Could you check a few things on this model? Use its own coordinates, in mm. Face numbers are marked on the shaded views. A direction names the side the tool comes from. Coordinates: 2 decimals unless noted, no trailing zeros. Loops run counter-clockwise (first coordinate to the right, second up) from the corner with the lowest first, then second, coordinate; pieces in that order, holes last. Notation, with made-up numbers: (55.25, 46) -> (96.25, 46) arc R35 ccw to (96.25, 85) -> close; hole circle Ø6 at (56.5, -32.5). An arc over 180 degrees is marked (long way). One line per question, with ' | ' between items.
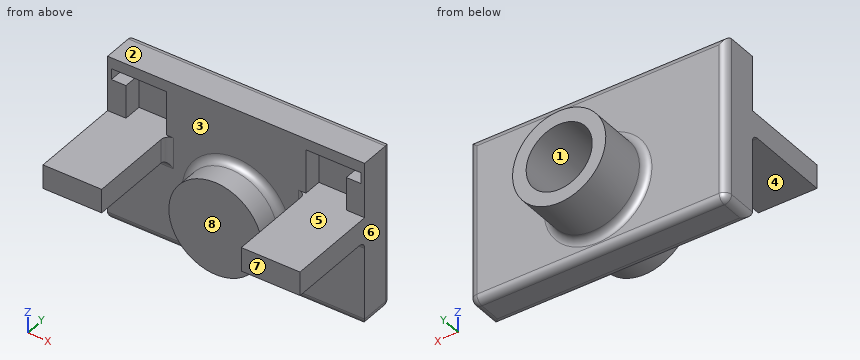
from build123d import *

# Parameters (mm, degrees)
SKETCH1_W           = 70
SKETCH1_H           = 45
BOSS_EXTRUDE1_DEPTH = 10
CUT_EXTRUDE1_DEPTH  = 5
FILLET1_R           = 2
SKETCH3_R           = 9
CUT_EXTRUDE3_DEPTH  = 25
BOSS_EXTRUDE2_START = 15
SKETCH5_R           = 12.7
SKETCH5_R_2         = 9
BOSS_EXTRUDE2_DEPTH = 15
FILLET2_R           = 2
SKETCH6_R           = 12.7
BOSS_EXTRUDE3_DEPTH = 8
FILLET3_R           = 2
SKETCH7_R           = 9
CUT_EXTRUDE4_DEPTH  = 5
SKETCH8_W           = 16
SKETCH8_H           = 6.5
BOSS_EXTRUDE4_DEPTH = 25
FILLET4_R           = 2


with BuildPart() as part:
    # Sketch1 → Boss-Extrude1 (new body)
    with BuildSketch(Plane(origin=(0, 0, 0), x_dir=(1, 0, 0), z_dir=(0, 1, 0))):
        with Locations((-1.479524439, -4.65323646)):
            Rectangle(SKETCH1_W, SKETCH1_H)
    extrude(amount=BOSS_EXTRUDE1_DEPTH)

    # Sketch2 → Cut-Extrude1 (cut)
    with BuildSketch(Plane.XZ):
        Polygon((28.520475561, 24.15323646), (17.520475561, 24.15323646), (17.520475561, 12.15323646), (28.520475561, 12.15323646), (28.520475561, 21.15323646), (32.520475561, 21.15323646), (32.520475561, 24.15323646), align=None)
        Polygon((-31.479524439, 21.15323646), (-35.479524439, 21.15323646), (-35.479524439, 24.15323646), (-31.479524439, 24.15323646), (-20.479524439, 24.15323646), (-20.479524439, 12.15323646), (-31.479524439, 12.15323646), align=None)
    extrude(amount=-CUT_EXTRUDE1_DEPTH, mode=Mode.SUBTRACT)

    # Fillet1
    fillet1_edges = [part.edges().sort_by_distance(p)[0] for p in [
        (33.520475561, 10, 4.65323646),
        (-1.479524439, 10, -17.84676354),
        (-36.479524439, 10, 4.65323646),
        (-1.479524439, 0, -17.84676354),
        (-36.479524439, 5, -17.84676354),
        (33.520475561, 5, -17.84676354),
        (-1.479524439, 10, 27.15323646),
    ]]
    fillet(fillet1_edges, radius=FILLET1_R)

    # Sketch3 → Cut-Extrude3 (cut)
    with BuildSketch(Plane(origin=(0, 10, 0), x_dir=(1, 0, 0), z_dir=(0, 1, 0))):
        with Locations(Location((-1.479524439, 0.84676354, 0), (0, 0, 270))):
            Circle(SKETCH3_R)
    extrude(amount=-CUT_EXTRUDE3_DEPTH, mode=Mode.SUBTRACT)

    # Sketch5 → Boss-Extrude2 (add)
    with BuildSketch(Plane(origin=(0, 10, 0), x_dir=(1, 0, 0), z_dir=(0, 1, 0)).offset(BOSS_EXTRUDE2_START)):
        with Locations(Location((-1.479524439, 0.84676354, 0), (0, 0, 270))):
            Circle(SKETCH5_R)
        with Locations(Location((-1.479524439, 0.84676354, 0), (0, 0, 270))):
            Circle(SKETCH5_R_2, mode=Mode.SUBTRACT)
    extrude(amount=-BOSS_EXTRUDE2_DEPTH)

    # Fillet2
    fillet2_edges = [part.edges().sort_by_distance(p)[0] for p in [
        (-1.479524439, 10, -13.54676354),
    ]]
    fillet(fillet2_edges, radius=FILLET2_R)

    # Sketch6 → Boss-Extrude3 (add)
    with BuildSketch(Plane.XZ):
        with Locations(Location((-1.479524439, -0.84676354, 0), (0, 0, 90))):
            Circle(SKETCH6_R)
    extrude(amount=BOSS_EXTRUDE3_DEPTH)

    # Fillet3
    fillet3_edges = [part.edges().sort_by_distance(p)[0] for p in [
        (-1.479524439, 0, -13.54676354),
    ]]
    fillet(fillet3_edges, radius=FILLET3_R)

    # Sketch7 → Cut-Extrude4 (cut)
    with BuildSketch(Plane(origin=(0, 0, 0), x_dir=(1, 0, 0), z_dir=(0, 1, 0))):
        with Locations(Location((-1.479524439, 0.84676354, 0), (0, 0, 270))):
            Circle(SKETCH7_R)
    extrude(amount=-CUT_EXTRUDE4_DEPTH, mode=Mode.SUBTRACT)

    # Sketch8 → Boss-Extrude4 (add)
    with BuildSketch(Plane.XZ):
        with Locations((-28.479524439, 8.90323646)):
            Rectangle(SKETCH8_W, SKETCH8_H)
        with Locations((25.520475561, 8.90323646)):
            Rectangle(SKETCH8_W, SKETCH8_H)
    extrude(amount=BOSS_EXTRUDE4_DEPTH)

    # Fillet4
    fillet4_edges = [part.edges().sort_by_distance(p)[0] for p in [
        (-20.479524439, 0, 8.90323646),
        (-28.479524439, 0, 5.65323646),
        (17.520475561, 0, 8.90323646),
        (25.520475561, 0, 5.65323646),
    ]]
    fillet(fillet4_edges, radius=FILLET4_R)


solid = part.part
1) I need wall thicknesses on line 1 along Z through (x, y) = (-21, 2.5); line 2 along Y through (x, z) = (-33, 10); line 3 along X through (y, z) = (-4, -8). Which ranges of each line are inside material? Lowest first, please. Write a range as from..to.
Data:
line 1: -17.85..12.15, 24.15..27.15 | line 2: -25..10 | line 3: -11.97..-6.94, 3.98..9.01
2) If we section it at A-A on y = -16: Please give me the cut outline in (x, z), and give its area (3 significant figures).
Data:
outline: (-36.48, 5.65) -> (-20.48, 5.65) -> (-20.48, 12.15) -> (-36.48, 12.15) -> close; (17.52, 5.65) -> (33.52, 5.65) -> (33.52, 12.15) -> (17.52, 12.15) -> close | area: 208 mm²
3) If we section it at C-C on z = 17.5: Please give me the cut outline in (x, y).
Data:
outline: (-36.48, 0) -> (-31.48, 0) -> (-31.48, 5) -> (-20.48, 5) -> (-20.48, 0) -> (17.52, 0) -> (17.52, 5) -> (28.52, 5) -> (28.52, 0) -> (33.52, 0) -> (33.52, 8) arc R2 ccw to (31.52, 10) -> (-34.48, 10) arc R2 ccw to (-36.48, 8) -> close
4) We'd pull the mould along Z, two halves only. Please class the marked faces 1, 2 and 3: pulls with the +Z half, pulls with the -Z half, needs draft (parallel to the pull), parting line crosses it, or undercut.
Data:
face 1: undercut | face 2: pulls with the +Z half | face 3: needs draft
5) If we section it at D-D on y = 16.5: Please give me the cut outline in (x, z), and give its area (3 significant figures).
Data:
outline: circle Ø25.4 at (-1.48, -0.85); hole circle Ø18 at (-1.48, -0.85) | area: 252 mm²
6) If we section it at B-B on x = -30: Please give me the cut outline in (y, z).
Data:
outline: (-25, 5.65) -> (-2, 5.65) arc R2 cw to (0, 3.65) -> (0, -15.85) arc R2 ccw to (2, -17.85) -> (8, -17.85) arc R2 ccw to (10, -15.85) -> (10, 25.15) arc R2 ccw to (8, 27.15) -> (0, 27.15) -> (0, 24.15) -> (5, 24.15) -> (5, 12.15) -> (-25, 12.15) -> close
7) On a 3-axis mill with a long thin cutter (end or side, diameter ignored), from which of +Z, -Z, +X, -X, +Y, -Y can I reach the whole of each face in a straight line? I mean the marked faces 4, 5, 6, 7 and 8. Say none if no direction works.
Data:
face 4: -Z, -X, -Y | face 5: -Y | face 6: +Z, -Z, +X, +Y, -Y | face 7: +Z, -Z, +X, -X, -Y | face 8: +Z, -Z, -Y
8) I'm going to push flat-ended pins straight in: pin 1 Ø1.5 at (x, z) = (-23.5, 0.5) entering from +Y; pin 2 Ø3.5 at (x, z) = (-25, 21) entering from -Y; pin 3 Ø3 at (x, y) = (16.5, -13.5) entering from -Z. Where does each tip first touch, or does it pass through?
Data:
pin 1: y = 10 | pin 2: y = 5 | pin 3: z = 5.65
